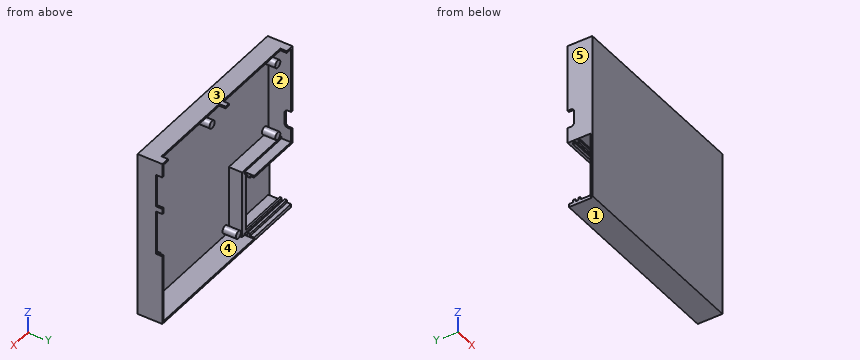
Autodesk Inventor part; units mm, degrees
ref_plane "YZ Plane" through (0, 0, 0) normal (1, 0, 0) x (0, 1, 0)
ref_plane "XZ Plane" through (0, 0, 0) normal (0, 1, 0) x (-1, 0, 0)
ref_plane "XY Plane" through (0, 0, 0) normal (0, 0, 1) x (1, 0, 0)
sketch "Sketch1" plane through (0, 0, 0) normal (0, 1, 0) x (-1, 0, 0)
  line L0 (0, 0) -> (102, 0)
  line L1 (102, 0) -> (102, -88)
  line L2 (102, -88) -> (0, -88)
  line L3 (0, -88) -> (0, 0)
  dimension "d0" = 102
  dimension "d1" = 88
extrude "Extrusion1" add sketch "Sketch1" along normal blind 1
sketch "Sketch3" plane through (0, 1, 0) normal (0, 1, 0) x (1, 0, 0)
  line L0 (0, 88) -> (-102, 88)
  line L1 (-102, 0) -> (0, 0)
  line L2 (-102, 88) -> (0, 88)
  line L3 (0, 88) -> (0, 0)
  line L4 (0, 0) -> (-102, 0)
  line L5 (-102, 0) -> (-102, 88)
  line L6 (-1, 1) -> (-1, 87)
  line L7 (-1, 87) -> (-101, 87)
  line L8 (-101, 87) -> (-101, 1)
  line L9 (-101, 1) -> (-1, 1)
  dimension "d7" = 1
extrude "Extrusion3" add sketch "Sketch3" along normal blind 12
sketch "Sketch4" plane through (-102, 0, 0) normal (0, 0, 1) x (1, 0, 0)
  line L0 (101, 13) -> (1, 13)
  line L1 (4.398, 13) -> (49.698, 13)
  line L2 (49.698, 13) -> (49.698, 9.6)
  line L3 (49.698, 9.6) -> (4.398, 9.6)
  line L4 (4.398, 9.6) -> (4.398, 13)
  line L5 (52.298, 13) -> (97.598, 13)
  line L6 (97.598, 13) -> (97.598, 9.6)
  line L7 (97.598, 9.6) -> (52.298, 9.6)
  line L8 (52.298, 9.6) -> (52.298, 13)
  line L9 (102, 0) -> (102, 13)
  line L10 (0, 0) -> (102, 0)
  dimension "d10" = 45.3
  dimension "d11" = 4.402
  dimension "d12" = 2.6
  dimension "d13" = 9.6
extrude "Extrusion4" cut sketch "Sketch4" against normal up to surface (1 mm away)
sketch "Sketch5" plane through (0, 0, 0) normal (1, 0, 0) x (0, 0, -1)
  line L0 (7.371, 13) -> (24.671, 13)
  line L1 (24.671, 13) -> (24.671, 9.6)
  line L2 (24.671, 9.6) -> (7.371, 9.6)
  line L3 (7.371, 9.6) -> (7.371, 13)
  line L4 (27.5, 13) -> (50.8, 13)
  line L5 (50.8, 13) -> (50.8, 9.6)
  line L6 (50.8, 9.6) -> (27.5, 9.6)
  line L7 (27.5, 9.6) -> (27.5, 13)
  line L8 (0, 13) -> (88, 13)
  line L9 (0, 0) -> (88, 0)
  line L10 (0, 13) -> (0, 9.6)
  dimension "d16" = 17.3
  dimension "d17" = 23.3
  dimension "d19" = 7.371
  dimension "d20" = 2.829
extrude "Extrusion5" cut sketch "Sketch5" against normal up to surface (1 mm away)
sketch "Sketch6" plane through (-102, 0, -88) normal (-1, 0, 0) x (0, 0, 1)
  line L0 (44.58, 11.3) -> (50.68, 11.3) construction
  line L1 (44.58, 9.6) -> (50.68, 9.6)
  arc A0 (42.88, 11.3) -> (44.58, 9.6) centre (44.58, 11.3) ccw
  arc A1 (50.68, 9.6) -> (52.38, 11.3) centre (50.68, 11.3) ccw
  line L2 (87, 1) -> (87, 13)
  line L3 (0, 0) -> (88, 0)
  line L4 (0, 13) -> (88, 13)
  line L5 (87, 13) -> (1, 13)
  line L6 (42.88, 13) -> (42.88, 11.3)
  line L7 (52.38, 11.3) -> (52.38, 13)
  line L8 (60.5, 9.6) -> (37.2, 9.6)
  line L9 (42.88, 13) -> (52.38, 13)
  point P0 (47.63, 11.3)
  dimension "d24" = 39.37
  dimension "d25" = 9.5
  dimension "d50" = 1.7
  dimension "d51" = 1.7
  dimension "d52" = 1.7
  dimension "d53" = 1.7
extrude "Extrusion6" cut sketch "Sketch6" against normal up to surface (1 mm away)
sketch "Sketch7" plane through (-102, 0, -88) normal (-1, 0, 0) x (0, 0, 1)
  line L0 (1, 1) -> (87, 1)
  line L1 (0, 13) -> (34.7, 13)
  line L2 (34.7, 13) -> (34.7, 1)
  line L3 (34.7, 1) -> (0, 1)
  line L4 (0, 1) -> (0, 13)
  line L5 (0, 13) -> (88, 13)
  line L6 (0, 0) -> (0, 13)
  point P0 (88, 0)
  dimension "d30" = 34.7
extrude "Extrusion7" cut sketch "Sketch7" against normal up to surface (1 mm away)
sketch "Sketch8" plane through (0, 1, 0) normal (0, 1, 0) x (1, 0, 0)
  line L0 (-101, 54.3) -> (-73, 54.3)
  line L1 (-70, 53.4922) -> (-70, 51.3)
  line L2 (-70, 51.3) -> (-101, 51.3)
  line L3 (-101, 51.3) -> (-101, 54.3)
  line L4 (-1, 87) -> (-101, 87)
  line L5 (-73, 54.3) -> (-73, 85)
  line L6 (-73, 87) -> (-70, 87)
  line L7 (-70, 87) -> (-70, 53.4922)
  line L8 (-101, 53.3) -> (-101, 1)
  line L9 (-102, 53.3) -> (-101, 53.3)
  line L10 (-73, 87) -> (-101, 87)
  line L11 (-101, 87) -> (-101, 85)
  line L12 (-101, 85) -> (-73, 85)
  point P0 (0, 0)
  dimension "d33" = 3
  dimension "d34" = 3
  dimension "d38" = 31
  dimension "d39" = 2
  dimension "d40" = 2
extrude "Extrusion8" add sketch "Sketch8" along normal blind 7
sketch "Sketch9" plane through (0, 8, 0) normal (0, 1, 0) x (1, 0, 0)
  line L0 (-101, 53.3) -> (-72, 53.3)
  line L1 (-72, 53.3) -> (-72, 52.3)
  line L2 (-72, 52.3) -> (-101, 52.3)
  line L3 (-101, 52.3) -> (-101, 53.3)
  line L4 (-73, 54.3) -> (-101, 54.3)
  line L5 (-101, 51.3) -> (-70, 51.3)
  line L6 (-101, 85) -> (-101, 88)
  line L7 (-101, 87) -> (-72, 87)
  line L8 (-72, 87) -> (-72, 86.3)
  line L9 (-72, 86.3) -> (-101, 86.3)
  line L10 (-101, 86.3) -> (-101, 87)
  line L11 (-101, 87) -> (-70, 87)
  line L12 (-73, 85) -> (-73, 54.3)
  point P0 (0, 0)
  point P1 (-101, 86.3)
  dimension "d41" = 1
  dimension "d42" = 1
  dimension "d45" = 0.7
  dimension "d46" = 1
extrude "Extrusion9" add sketch "Sketch9" along normal up to surface (5 mm away)
sketch "Sketch10" plane through (-101, 1, -54.3) normal (-1, 0, 0) x (0, 0, 1)
  line L0 (1, 0) -> (1, 7)
  line L1 (53.3, 0) -> (-32.7, 0)
  line L2 (1, 6) -> (-32, 6)
  line L3 (-32, 6) -> (-32, 0)
  line L4 (-32, 0) -> (1, 0)
  line L5 (1, 0) -> (1, 6)
  line L6 (-32, 7) -> (-32, 12)
  line L7 (-30.7, 7) -> (0, 7)
  point P0 (54.3, -1)
  point P1 (1, 10)
  dimension "d47" = 1
extrude "Extrusion10" cut sketch "Sketch10" against normal up to surface (28 mm away)
sketch "Sketch11" plane through (-101, 8, -54.3) normal (-1, 0, 0) x (0, 0, 1)
  line L0 (1, 5) -> (1, -7)
  line L1 (1, 1.6) -> (0, 1.6)
  line L2 (0, 1.6) -> (0, 2.9)
  line L3 (0, 2.9) -> (1, 2.9)
  line L4 (1, 2.9) -> (1, 1.6)
  line L5 (-32, 0) -> (-32, 5)
  line L6 (-32, 1.6) -> (-30.7, 1.6)
  line L7 (-30.7, 1.6) -> (-30.7, 2.9)
  line L8 (-30.7, 2.9) -> (-32, 2.9)
  line L9 (-32, 2.9) -> (-32, 1.6)
  line L10 (-32, 0) -> (-30.7, 0)
  line L11 (-30.7, -1) -> (-30.7, 0)
  line L12 (0, -1) -> (0, 0)
  point P0 (54.3, -8)
  point P1 (1, 2.9)
  point P2 (-32, 2.9)
  dimension "d54" = 1.6
extrude "Extrusion11" add sketch "Sketch11" against normal up to surface (29 mm away)
sketch "Sketch12" plane through (0, 1, 0) normal (0, 1, 0) x (1, 0, 0)
  circle A0 centre (-98, 9.46) radius 2
  circle A1 centre (-98, 49) radius 2
  circle A2 centre (-46.5, 9.94) radius 2
  circle A3 centre (-67.111, 83.775) radius 2
  circle A4 centre (-4.51, 83.775) radius 2
  circle A5 centre (-4.39, 55.98) radius 2
  line L0 (-49.702, 1) -> (-4.402, 1)
  line L1 (-1, 7.371) -> (-1, 1)
  line L2 (-1, 1) -> (-4.402, 1)
  line L3 (-1, 87) -> (-1, 50.8)
  point P0 (0, 0)
  dimension "d57" = 8.94
  dimension "d58" = 45.5
  dimension "d59" = 4
  dimension "d60" = 54.98
  dimension "d61" = 3.39
  dimension "d62" = 3.51
  dimension "d63" = 82.775
  dimension "d64" = 82.775
  dimension "d65" = 66.111
  dimension "d66" = 97
  dimension "d67" = 8.46
  dimension "d68" = 48
  dimension "d69" = 97
extrude "Extrusion12" add sketch "Sketch12" along normal up to surface (7 mm away)
properties part number "BaseCase"
Model file for the job. Use its own axes, mm. Face numbers are marked on the shaded views. A direction names the side the tool comes from. Give positions to 0.01 mm unless a question says otherwise; leave off trailing zeros. Write each loop counter-clockwise with the first axis right and the second up, starting at its lowest first coordinate (ties: lowest second). Pieces come first, ordered by that corner, then holes. Notation, with made-up numbers: (-19, -23.5) - (-3, -23.5) arc R35 cw to (-3, 8.5) - close; hole circle Ø7 at (61, 68). An arc over 180 degrees is marked (long way). Answer as CSV lines item,"result".
1. Pin check, flat tips, straight feed: pin 1 (1 mm diameter, centred on y = 2.5, z = -11, fed in from +X); pin 2 (1 mm diameter, centred on x = -91.5, y = 10.5, fed in from +Z); pin 3 (1.1 mm diameter, centred on x = -71.5, z = -0.5, fed in from +Y); pin 4 (3 mm diameter, centred on x = -26, z = -77, fed in from +Y). Stop position of each tip, or through.
Responses:
pin 1,"stops at x = 0"
pin 2,"stops at z = -52.3"
pin 3,"stops at y = 9.6"
pin 4,"stops at y = 1"
2. Band-saw the part on A-A (y = 4.75). Write the cut outline in (x, z) (3 decimals), and give its area (3 significant figures).
Responses:
outline,"(-102, -53.3) - (-73, -53.3) - (-73, -86.3) - (-101, -86.3) - (-101, -88) - (0, -88) - (0, 0) - (-102, 0) - close; circle Ø4 at (-98, -49); circle Ø4 at (-98, -9.46); circle Ø4 at (-67.111, -83.775); circle Ø4 at (-46.5, -9.94); circle Ø4 at (-4.51, -83.775); circle Ø4 at (-4.39, -55.98); hole (-101, -51.3) - (-70, -51.3) - (-70, -87) - (-1, -87) - (-1, -1) - (-101, -1) - close"
area,"599 mm2"
3. Band-saw the part on D-D (z = -55.98). Write the cut outline in (x, y).
Responses:
outline,"(-102, 0) - (0, 0) - (0, 13) - (-1, 13) - (-1, 1) - (-2.39, 1) - (-2.39, 8) - (-6.39, 8) - (-6.39, 1) - (-70, 1) - (-70, 8) - (-73, 8) - (-73, 1) - (-102, 1) - close"
4. Band-saw the part on B-B (z = -76). Write the cut outline in (x, y), and give its area (3 significant figures).
Responses:
outline,"(-102, 0) - (0, 0) - (0, 13) - (-1, 13) - (-1, 1) - (-70, 1) - (-70, 8) - (-73, 8) - (-73, 1) - (-102, 1) - close"
area,"135 mm2"
5. Drill centre lines: L1, parallel to Z at x = -81, y = 3; L2, parallel to Z at x = -89, y = 9; L3, parallel to Z at x = -17.5, y = 6.5. Where is each one in solid material? Low to high. Write a range as [from, to].
Responses:
L1,"z = [-88, -86.3], [-53.3, -51.3], [-1, 0]"
L2,"z = [-88, -86.3], [-53.3, -52.3], [-1, 0]"
L3,"z = [-88, -87], [-1, 0]"
6. 3-axis set-ups, long thin cutter, end or side, ignore diameter. For the marked faces 4 and 5: which of +Z, -Z, +X, -X, +Y, -Y reach the whole face in a straight line?
Responses:
face 4,"+Y"
face 5,"+Z, -Z, -X, +Y, -Y"
7. Two-plate mould, pull along Z, no slides. Class the marked faces 1, 2 and 3: +Z half, -Z half, draft (parallel to the pull), parting line (faces both ways), or undercut.
Responses:
face 1,"-Z half"
face 2,"undercut"
face 3,"+Z half"
